```python
from build123d import *

# Parameters (mm, degrees)
CROQUIS1_W                       = 580
CROQUIS1_H                       = 8.5
CROQUIS4_R                       = 9.75
SALIENTE_EXTRUIR1_DEPTH          = 4
MATRIZL1_COUNT                   = 2
MATRIZL1_PITCH                   = 442
SALIENTE_EXTRUIR3_DEPTH          = 3.8
MATRIZL2_COUNT                   = 2
MATRIZL2_PITCH                   = 40
MATRIZL3_COUNT                   = 2
MATRIZL3_PITCH                   = 332
MATRIZL3_COPY_1_DEPTH            = 3.8
CROQUIS6_R                       = 8.5
SALIENTE_EXTRUIR4_DEPTH          = 3.8
MATRIZL4_COUNT                   = 2
MATRIZL4_PITCH                   = 40
MATRIZL5_COUNT                   = 2
MATRIZL5_PITCH                   = 110
MATRIZL5_COPY_1_SKETCH_R         = 8.5
MATRIZL5_COPY_1_DEPTH            = 3.8
CROQUIS8_R                       = 10
CORTAR_EXTRUIR1_DEPTH            = 36
CROQUIS9_R                       = 9.75
SALIENTE_EXTRUIR5_DEPTH          = 4
CROQUIS10_R                      = 8.5
SALIENTE_EXTRUIR6_DEPTH          = 8
CHAFL_N1_SIZE                    = 1
SALIENTE_EXTRUIR7_DEPTH          = 5
SALIENTE_EXTRUIR7_DEPTH_BACK     = 5
CROQUIS12_R                      = 15
CROQUIS13_W                      = 6
CROQUIS13_H                      = 3.35
SALIENTE_EXTRUIR8_DEPTH          = 40
CORTAR_EXTRUIR2_START            = -81
CROQUIS15_R                      = 35.701734295
CORTAR_EXTRUIR2_DEPTH            = 81
TALADRO_DE_MARGEN_PARA_M71_D     = 7.6
TALADRO_DE_MARGEN_PARA_M71_DEPTH = 30
TALADRO_DE_MARGEN_PARA_M71_TIP   = 2.283270352


with BuildPart() as part:
    # Croquis1 → Revolución1 (revolve)
    with BuildSketch(Plane.XY, mode=Mode.PRIVATE) as revoluci_n1_sk:
        with Locations((290, 4.25)):
            Rectangle(CROQUIS1_W, CROQUIS1_H)
    revolve(revoluci_n1_sk.sketch.rotate(Axis((0, 8.5, 0), (1, 0, 0)), 270), axis=Axis((0, 8.5, 0), (1, 0, 0)))

    # Croquis4 → Saliente-Extruir1 (add)
    with BuildSketch(Plane(origin=(580, 0, 0), x_dir=(0, 0, -1), z_dir=(1, 0, 0))):
        with Locations((0, 8.5)):
            Circle(CROQUIS4_R)
    saliente_extruir1 = extrude(amount=-SALIENTE_EXTRUIR1_DEPTH)

    # MatrizL1: Saliente-Extruir1 ×2
    with Locations(*[(-i * MATRIZL1_PITCH, 0, 0) for i in range(1, MATRIZL1_COUNT)]):
        add(saliente_extruir1)

    # Croquis5 → Saliente-Extruir3 (add, symmetric)
    with BuildSketch(Plane(origin=(162.25, 0, 0), x_dir=(0, 0, -1), z_dir=(1, 0, 0))):
        with BuildLine():
            ThreePointArc((-8.57686354, 11.227161863), (0, -0.5), (8.57686354, 11.227161863))
            ThreePointArc((8.57686354, 11.227161863), (6.71423124, 16.165722115), (4.341375372, 20.880415264))
            ThreePointArc((4.341375372, 20.880415264), (0, 23.4), (-4.341375372, 20.880415264))
            ThreePointArc((-4.341375372, 20.880415264), (-6.71423124, 16.165722115), (-8.57686354, 11.227161863))
        make_face()
    saliente_extruir3 = extrude(amount=SALIENTE_EXTRUIR3_DEPTH, both=True)

    # MatrizL2: Saliente-Extruir3 ×2
    with Locations(*[(i * MATRIZL2_PITCH, 0, 0) for i in range(1, MATRIZL2_COUNT)]):
        add(saliente_extruir3)

    # MatrizL3: Saliente-Extruir3 ×2
    with Locations(*[(i * MATRIZL3_PITCH, 0, 0) for i in range(1, MATRIZL3_COUNT)]):
        add(saliente_extruir3)

    # MatrizL3 copy 1 sketch → MatrizL3 copy 1 (add, symmetric)
    with BuildSketch(Plane(origin=(534.25, 0, 0), x_dir=(0, 0, -1), z_dir=(1, 0, 0))):
        with BuildLine():
            ThreePointArc((-8.57686354, 11.227161863), (0, -0.5), (8.57686354, 11.227161863))
            ThreePointArc((8.57686354, 11.227161863), (6.71423124, 16.165722115), (4.341375372, 20.880415264))
            ThreePointArc((4.341375372, 20.880415264), (0, 23.4), (-4.341375372, 20.880415264))
            ThreePointArc((-4.341375372, 20.880415264), (-6.71423124, 16.165722115), (-8.57686354, 11.227161863))
        make_face()
    extrude(amount=MATRIZL3_COPY_1_DEPTH, both=True)

    # Croquis6 → Saliente-Extruir4 (add, symmetric)
    with BuildSketch(Plane(origin=(272.25, 0, 0), x_dir=(0, 0, -1), z_dir=(1, 0, 0))):
        with BuildLine():
            ThreePointArc((-12.722376543, 12.627249768), (-14.9, 8.5), (-12.722376543, 4.372750232))
            ThreePointArc((-12.722376543, 4.372750232), (-8.363270987, 1.70804262), (-3.754994824, -0.497917196))
            ThreePointArc((-3.754994824, -0.497917196), (9.75, 8.5), (-3.754994824, 17.497917196))
            ThreePointArc((-3.754994824, 17.497917196), (-8.363270987, 15.29195738), (-12.722376543, 12.627249768))
        make_face()
        with Locations(Location((0, 8.5, 0), (0, 0, 180))):
            Circle(CROQUIS6_R, mode=Mode.SUBTRACT)
    saliente_extruir4 = extrude(amount=SALIENTE_EXTRUIR4_DEPTH, both=True)

    # MatrizL4: Saliente-Extruir4 ×2
    with Locations(*[(i * MATRIZL4_PITCH, 0, 0) for i in range(1, MATRIZL4_COUNT)]):
        add(saliente_extruir4)

    # MatrizL5: Saliente-Extruir4 ×2
    with Locations(*[(i * MATRIZL5_PITCH, 0, 0) for i in range(1, MATRIZL5_COUNT)]):
        add(saliente_extruir4)

    # MatrizL5 copy 1 sketch → MatrizL5 copy 1 (add, symmetric)
    with BuildSketch(Plane(origin=(422.25, 0, 0), x_dir=(0, 0, -1), z_dir=(1, 0, 0))):
        with BuildLine():
            ThreePointArc((-12.722376543, 12.627249768), (-14.9, 8.5), (-12.722376543, 4.372750232))
            ThreePointArc((-12.722376543, 4.372750232), (-8.363270987, 1.70804262), (-3.754994824, -0.497917196))
            ThreePointArc((-3.754994824, -0.497917196), (9.75, 8.5), (-3.754994824, 17.497917196))
            ThreePointArc((-3.754994824, 17.497917196), (-8.363270987, 15.29195738), (-12.722376543, 12.627249768))
        make_face()
        with Locations(Location((0, 8.5, 0), (0, 0, 180))):
            Circle(MATRIZL5_COPY_1_SKETCH_R, mode=Mode.SUBTRACT)
    extrude(amount=MATRIZL5_COPY_1_DEPTH, both=True)

    # Croquis8 → Cortar-Extruir1 (cut)
    with BuildSketch(Plane(origin=(564, 0, 0), x_dir=(0, 0, -1), z_dir=(1, 0, 0))):
        with Locations((0, 8.5)):
            Circle(CROQUIS8_R)
    extrude(amount=CORTAR_EXTRUIR1_DEPTH, mode=Mode.SUBTRACT)

    # Croquis9 → Saliente-Extruir5 (add)
    with BuildSketch(Plane(origin=(564, 0, 0), x_dir=(0, 0, -1), z_dir=(1, 0, 0))):
        with Locations((0, 8.5)):
            Circle(CROQUIS9_R)
    extrude(amount=-SALIENTE_EXTRUIR5_DEPTH)


with BuildPart() as body_2:
    # Simetría1: mirrored copy
    add(part.part.mirror(Plane.ZY))

    # Croquis10 → Saliente-Extruir6 (add)
    with BuildSketch(Plane.ZY.offset(564)):
        with Locations((0, 8.5)):
            Circle(CROQUIS10_R)
    extrude(amount=SALIENTE_EXTRUIR6_DEPTH)

    # Chaflán1
    chafl_n1_edges = [body_2.edges().sort_by_distance(p)[0] for p in [
        (-572, 8.5, -8.5),
    ]]
    chamfer(chafl_n1_edges, length=CHAFL_N1_SIZE)

    # Croquis12 → Saliente-Extruir7 (add, two sides: drawn at the far end of the back side and taken through both)
    with BuildSketch(Plane(origin=(-113, 0, 0), x_dir=(0, 0, -1), z_dir=(1, 0, 0)).offset(-SALIENTE_EXTRUIR7_DEPTH_BACK)):
        with Locations((0, 8.5)):
            Circle(CROQUIS12_R)
    extrude(amount=SALIENTE_EXTRUIR7_DEPTH + SALIENTE_EXTRUIR7_DEPTH_BACK)

    # Croquis13 → Saliente-Extruir8 (add)
    with BuildSketch(Plane(origin=(-108, 0, 0), x_dir=(0, 0, -1), z_dir=(1, 0, 0))):
        with Locations((0, 18.12798686)):
            Rectangle(CROQUIS13_W, CROQUIS13_H)
    extrude(amount=SALIENTE_EXTRUIR8_DEPTH)

    # Croquis15 → Cortar-Extruir2 (cut)
    with BuildSketch(Plane(origin=(0, 0, 0), x_dir=(0, 0, -1), z_dir=(1, 0, 0)).offset(CORTAR_EXTRUIR2_START)):
        with Locations((0, 8.5)):
            Circle(CROQUIS15_R)
    extrude(amount=CORTAR_EXTRUIR2_DEPTH, mode=Mode.SUBTRACT)

    # Taladro de margen para M71
    with Locations(Plane(origin=(-81, 8.5, 0), x_dir=(0, 0, 1), z_dir=(1, 0, 0))):
        with Locations((0, 0)):
            Hole(TALADRO_DE_MARGEN_PARA_M71_D / 2, depth=TALADRO_DE_MARGEN_PARA_M71_DEPTH)
            with Locations((0, 0, -(TALADRO_DE_MARGEN_PARA_M71_DEPTH + TALADRO_DE_MARGEN_PARA_M71_TIP / 2))):  # 118° drill point
                Cone(0, TALADRO_DE_MARGEN_PARA_M71_D / 2, TALADRO_DE_MARGEN_PARA_M71_TIP, mode=Mode.SUBTRACT)


solid = body_2.part
```
Geometry: final body of the model. Coordinates: model frame, mm. A direction names the side the tool comes from. Coordinates: 2 decimals unless noted, no trailing zeros. Order: outer loops, then holes, each group sorted by start corner. A loop starts at its lowest first (then second) coordinate and runs counter-clockwise, first axis right, second up. Notation, with made-up numbers: M 61.25,-2.5 L 95.25,-2.5 A8 cw 95.25,4.5 Z; hole C 27,47 d4. An arc over 180 degrees is marked long. Answer in a Markdown table with one row per item. Add a question column.
Q1. Mould query, pull axis Y, two halves, no side actions, for faces 1 (the cylindrical face through (-534.303, 16.098, -6.744)), 2 (the flat face through (-158.45, 18, 0)), 3 (the cylindrical face through (-96.21, 4.73, 0.49)), 4 (the cylindrical face through (-312.303, 8.232, -9.746)). Classes: released by +Y, released by -Y, zero draft, split by the parting line, or undercut.
Q2. Contact query for flat-ended pins moving along their axis: P1, Ø8, axis at y = -2.5, z = 1, coming from the -X side; P2, Ø6, axis at x = -264, z = -5.5, coming from the -Y side; P3, Ø1.7, axis at x = -88, y = 18.5, coming from the -Z side; P4, Ø5, axis at x = -98.5, z = 1, coming from the +Y side. Output: stop coordinate, or through.
Q3. Reachability of faces 5 (the cylindrical face through (-534.3, 23.4, -0.1)), 6 (the cylindrical face through (-562.03, -1.02, 2.11)), 7 (the flat face through (-572, 9, 0)), 8 (the flat face through (-138, 17.2, -0.7)), 9 (the cylindrical face through (-534.3, 16.2, 6.7)) from +Z, -Z, +X, -X, +Y, -Y: full face, straight path, thin tool, end or side. Return the list, or none.
Q4. Section query A-A on x = -511.5. Return the cut outline in (y, z), and give its area (3 significant figures).
Q5. Line query: L1, parallel to X at y = 20.5, z = 2.75; L2, parallel to Y at x = -95.5, z = 0; L3, parallel to X at y = 2.5, z = -9.5. Output: solid intervals per line, ascending.
Completed:
| question | item | result |
|---|---|---|
| 1 | face 1 | released by +Y |
| 1 | face 2 | zero draft |
| 1 | face 3 | undercut |
| 1 | face 4 | split by the parting line |
| 2 | P1 | stops at x = -572 |
| 2 | P2 | stops at y = 0.38 |
| 2 | P3 | stops at z = -3 |
| 2 | P4 | stops at y = 19.8 |
| 3 | face 5 | -X, +Y |
| 3 | face 6 | -X |
| 3 | face 7 | +Z, -Z, -X, +Y, -Y |
| 3 | face 8 | none |
| 3 | face 9 | +Z, +Y |
| 4 | outline | C 8.5,0 d17 |
| 4 | area | 227 mm2 |
| 5 | L1 | x = -538.05 to -530.45, -498.05 to -490.45, -206.05 to -198.45, -166.05 to -158.45, -118 to -108 |
| 5 | L2 | y = 0 to 4.7, 12.3 to 19.8 |
| 5 | L3 | x = -118 to -108 |
